Solid Edge part; units mm, degrees
sketch "Sketch1" plane through (0, 0, 0) normal (0, 0, 1) x (1, 0, 0)
  line L0 (250, -175) -> (-250, -175)
  line L1 (-250, -175) -> (-250, 175)
  line L2 (-250, 175) -> (250, 175)
  line L3 (250, 175) -> (250, -175)
extrude "Protrusion1" add sketch "Sketch1" along normal blind 30
chamfer "Chaflán_1" distance 50 angle 45 4 edges at (250, -175, 15) (-250, -175, 15) (250, 175, 15) (-250, 175, 15)
hole "Agujero_1" at (199.5, 22.5, 0) direction (0, 0, 1) diameter 6.647 end through all thread major 8 thread length 15
hole "Hole1" at (160.5, 22.5, 0) direction (0, 0, 1) diameter 6.647 end through all thread major 8 thread length 15
hole "Hole2" at (199.5, -22.5, 0) direction (0, 0, 1) diameter 6.647 end through all thread major 8 thread length 15
hole "Hole3" at (160.5, -22.5, 0) direction (0, 0, 1) diameter 6.647 end through all thread major 8 thread length 15
hole "Hole4" at (67.5, 109.5, 0) direction (0, 0, 1) diameter 6.647 end through all thread major 8 thread length 15
hole "Hole5" at (22.5, 109.5, 0) direction (0, 0, 1) diameter 6.647 end through all thread major 8 thread length 15
hole "Hole6" at (67.5, 70.5, 0) direction (0, 0, 1) diameter 6.647 end through all thread major 8 thread length 15
hole "Hole7" at (22.5, 70.5, 0) direction (0, 0, 1) diameter 6.647 end through all thread major 8 thread length 15
hole "Hole8" at (-22.5, 70.5, 0) direction (0, 0, 1) diameter 6.647 end through all thread major 8 thread length 15
hole "Hole9" at (-22.5, 109.5, 0) direction (0, 0, 1) diameter 6.647 end through all thread major 8 thread length 15
hole "Hole10" at (-67.5, 109.5, 0) direction (0, 0, 1) diameter 6.647 end through all thread major 8 thread length 15
hole "Hole11" at (-67.5, 70.5, 0) direction (0, 0, 1) diameter 6.647 end through all thread major 8 thread length 15
hole "Hole12" at (-160.5, 22.5, 0) direction (0, 0, 1) diameter 6.647 end through all thread major 8 thread length 15
hole "Hole13" at (-199.5, 22.5, 0) direction (0, 0, 1) diameter 6.647 end through all thread major 8 thread length 15
hole "Hole14" at (-160.5, -22.5, 0) direction (0, 0, 1) diameter 6.647 end through all thread major 8 thread length 15
hole "Hole15" at (-199.5, -22.5, 0) direction (0, 0, 1) diameter 6.647 end through all thread major 8 thread length 15
hole "Hole16" at (-67.5, -70.5, 0) direction (0, 0, 1) diameter 6.647 end through all thread major 8 thread length 15
hole "Hole17" at (-22.5, -70.5, 0) direction (0, 0, 1) diameter 6.647 end through all thread major 8 thread length 15
hole "Hole18" at (-22.5, -109.5, 0) direction (0, 0, 1) diameter 6.647 end through all thread major 8 thread length 15
hole "Hole19" at (-67.5, -109.5, 0) direction (0, 0, 1) diameter 6.647 end through all thread major 8 thread length 15
hole "Hole20" at (22.5, -109.5, 0) direction (0, 0, 1) diameter 6.647 end through all thread major 8 thread length 15
hole "Hole21" at (22.5, -70.5, 0) direction (0, 0, 1) diameter 6.647 end through all thread major 8 thread length 15
hole "Hole22" at (67.5, -70.5, 0) direction (0, 0, 1) diameter 6.647 end through all thread major 8 thread length 15
hole "Hole23" at (67.5, -109.5, 0) direction (0, 0, 1) diameter 6.647 end through all thread major 8 thread length 15
properties part number "1983-1100-001" material "Acero, estructural"
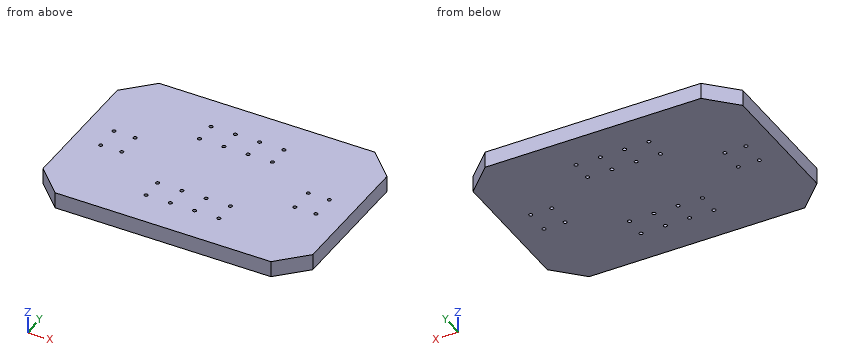
Source: CAD feature listing. Evaluate the final solid. Frame: model axes, mm. Give positions to 0.01 mm unless a question says otherwise; leave off trailing zeros. Loops run counter-clockwise (first coordinate to the right, second up) from the corner with the lowest first, then second, coordinate; pieces in that order, holes last. Notation, with made-up numbers: M 36.25,81 L 57.25,81 A37 cw 57.25,119 Z; hole C 73.5,25.25 d6. An arc over 180 degrees is marked long. Put each result on its own line as item: value.
Q1. Section B-B (x = 212). Return the cut outline in (y, z).
Response values:
outline: M -163,0 L 163,0 L 163,30 L -163,30 Z
Q2. Line query: probe 1 along Y at (x, z) = (-67.5, 17.75); probe 2 along X at (y, z) = (-109.5, 24.25); probe 3 along Y at (x, z) = (-160.5, 23). Output: solid intervals per line, ascending. Write a range as [from, to].
Response values:
probe 1: y = [-175, -112.82], [-106.18, -73.82], [-67.18, 67.18], [73.82, 106.18], [112.82, 175]
probe 2: x = [-250, -70.82], [-64.18, -25.82], [-19.18, 19.18], [25.82, 64.18], [70.82, 250]
probe 3: y = [-175, -25.82], [-19.18, 19.18], [25.82, 175]
Q3. Section A-A (z = 8.5). Count the separate pieces of the cut face and the enclosed holes in it, and give its area (3 significant figures).
Response values:
separate pieces: 1
enclosed holes: 24
area: 169,000 mm²
